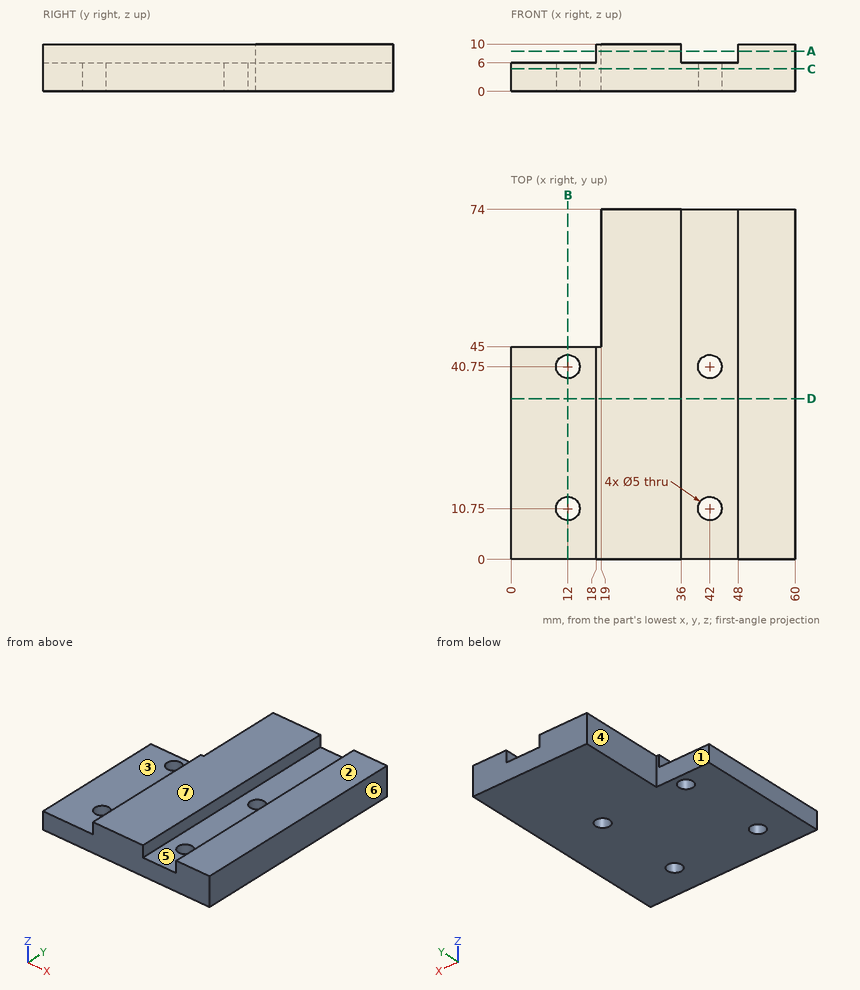
Input: dimensioned drawing with shaded views. Units: mm. Origin: part minimum x, y, z. A direction names the side the tool comes from. Give positions to 0.01 mm unless a question says otherwise; leave off trailing zeros. Write each loop counter-clockwise with the first axis right and the second up, starting at its lowest first coordinate (ties: lowest second). Pieces come first, ordered by that corner, then holes. Notation, with made-up numbers: (25.5, -21) - (76.5, -21) arc R26 ccw to (76.5, 4) - close; hole circle Ø8 at (56.25, 12.5). An arc over 180 degrees is marked (long way). Write item = value, one per line. Start each with the question number.
1) Draft query along X for the marked faces 4, 5, 6 and 7. Return one class per face: pulls with the +X half, pulls with the -X half, needs draft (parallel to the pull), parting line crosses it, or undercut.
2) Material intervals for L1, parallel to Y at x = 42, z = 2.3; L2, parallel to Y at x = 12, z = 3.05; L3, parallel to X at y = 23.5, z = 7.25, sorted ascending. Write a range as [from, to].
3) Cut plane A-A (z = 8.5). Return loops of the section in (x, y).
4) Pin query (flat end, axial travel): pin 1 (2 mm diameter, centred on y = 24.5, z = 9, fed in from -X); pin 2 (1 mm diameter, centred on x = 9, y = 44, fed in from +Z). Return the tip coordinate at first contact, or that it passes through.
5) Cut plane D-D (y = 34). Return loops of the section in (x, z), and give its area (3 significant figures).
6) Cut plane C-C (z = 4.75). Return loops of the section in (x, y), and give its area (3 significant figures).
7) Reachability of the marked faces 1, 2 and 3 from +Z, -Z, +X, -X, +Y, -Y: full face, straight path, thin tool, end or side. Return the list, or none.
8) Cut plane B-B (x = 12). Return loops of the section in (y, z).
Answers follow:
q1.face_4 = pulls with the -X half
q1.face_5 = undercut
q1.face_6 = pulls with the +X half
q1.face_7 = needs draft
q2.L1 = [0, 8.25], [13.25, 38.25], [43.25, 74]
q2.L2 = [0, 8.25], [13.25, 38.25], [43.25, 45]
q2.L3 = [18, 36], [48, 60]
q3.outline = (18, 0) - (36, 0) - (36, 74) - (19, 74) - (19, 45) - (18, 45) - close; (48, 0) - (60, 0) - (60, 74) - (48, 74) - close
q4.pin_1 = 18
q4.pin_2 = 6
q5.outline = (0, 0) - (60, 0) - (60, 10) - (48, 10) - (48, 6) - (36, 6) - (36, 10) - (18, 10) - (18, 6) - (0, 6) - close
q5.area = 480 mm^2
q6.outline = (0, 0) - (60, 0) - (60, 74) - (19, 74) - (19, 45) - (0, 45) - close; hole circle Ø5 at (12, 10.75); hole circle Ø5 at (12, 40.75); hole circle Ø5 at (42, 10.75); hole circle Ø5 at (42, 40.75)
q6.area = 3,810 mm^2
q7.face_1 = +Z, -Z, -X, +Y
q7.face_2 = +Z, +X, -X, +Y, -Y
q7.face_3 = +Z, -X, +Y, -Y
q8.outline = (0, 0) - (8.25, 0) - (8.25, 6) - (0, 6) - close; (13.25, 0) - (38.25, 0) - (38.25, 6) - (13.25, 6) - close; (43.25, 0) - (45, 0) - (45, 6) - (43.25, 6) - close
